from build123d import *

# Parameters (mm, degrees)
F0_R     = 3
F1_DEPTH = 3.95
F0_R_2   = 2.499
F2_DEPTH = 3.45
F3_R     = 3.69999
F4_R     = 3.7


# Not quite as in the source:
# - a fillet or chamfer is up to 0.001 mm smaller than in the source, because OpenCascade refuses the exact size


with BuildPart() as f1:
    # F0 (on Front) → F1 (new body, symmetric)
    with BuildSketch(Plane.XZ):
        Polygon((19.7, 0), (-19.7, 0), (-19.7, -23.4), (-12.3, -23.4), (-12.3, -7.4), (19.7, -7.4), align=None)
        with Locations((-16, -19.7)):
            Circle(F0_R, mode=Mode.SUBTRACT)
        with Locations((-16, -11.7)):
            Circle(F0_R, mode=Mode.SUBTRACT)
        with Locations((-16, -3.7)):
            Circle(F0_R, mode=Mode.SUBTRACT)
        with Locations((-8, -3.7)):
            Circle(F0_R, mode=Mode.SUBTRACT)
        with Locations((0, -3.7)):
            Circle(F0_R, mode=Mode.SUBTRACT)
        with Locations((8, -3.7)):
            Circle(F0_R, mode=Mode.SUBTRACT)
        with Locations((16, -3.7)):
            Circle(F0_R, mode=Mode.SUBTRACT)
    extrude(amount=F1_DEPTH, both=True)

    # F0 (on Front) → F2 (join, symmetric)
    with BuildSketch(Plane.XZ):
        with Locations((16, -3.7)):
            Circle(F0_R)
        with Locations((16, -3.7)):
            Circle(F0_R_2, mode=Mode.SUBTRACT)
        with Locations((8, -3.7)):
            Circle(F0_R)
        with Locations((8, -3.7)):
            Circle(F0_R_2, mode=Mode.SUBTRACT)
        with Locations((0, -3.7)):
            Circle(F0_R)
        with Locations((0, -3.7)):
            Circle(F0_R_2, mode=Mode.SUBTRACT)
        with Locations((-8, -3.7)):
            Circle(F0_R)
        with Locations((-8, -3.7)):
            Circle(F0_R_2, mode=Mode.SUBTRACT)
        with Locations((-16, -3.7)):
            Circle(F0_R)
        with Locations((-16, -3.7)):
            Circle(F0_R_2, mode=Mode.SUBTRACT)
        with Locations((-16, -19.7)):
            Circle(F0_R)
        with Locations((-16, -19.7)):
            Circle(F0_R_2, mode=Mode.SUBTRACT)
        with Locations((-16, -11.7)):
            Circle(F0_R)
        with Locations((-16, -11.7)):
            Circle(F0_R_2, mode=Mode.SUBTRACT)
    extrude(amount=F2_DEPTH, both=True)

    # F3 (radius 3.7 in the source; OpenCascade refuses exactly that, so slightly less here)
    f3_edges = [f1.edges().sort_by_distance(p)[0] for p in [
        (19.7, 0, 0),
        (19.7, 0, -7.4),
        (-12.3, 0, -23.4),
        (-19.7, 0, -23.4),
    ]]
    fillet(f3_edges, radius=F3_R)

    # F4
    f4_edges = [f1.edges().sort_by_distance(p)[0] for p in [
        (-19.7, 0, 0),
    ]]
    fillet(f4_edges, radius=F4_R)


solid = f1.part
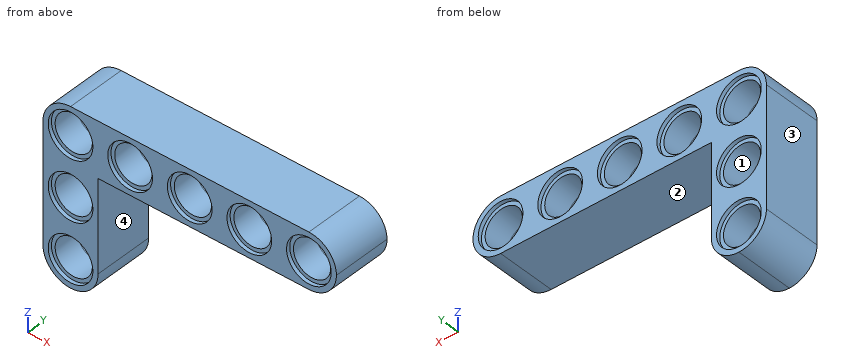
Could you check a few things on this model? Use its own coordinates, in mm. Face numbers are marked on the shaded views. Round coordinates to 2 decimals unless told otherwise and drop trailing zeros. Order: outer loops, then holes, each group sorted by start corner. A loop starts at its lowest first (then second) coordinate and runs counter-clockwise, first axis right, second up.
(1) I'm going to push flat-ended pins straight in: pin 1 (5.5 mm diameter, centred on x = -8, z = -3.7, fed in from +Y); pin 2 (1 mm diameter, centred on x = -6, y = 1, fed in from -Z); pin 3 (5.5 mm diameter, centred on x = -16, z = -19.7, fed in from -Y). Where does each tip first touch, or does it pass through?
Response values:
pin 1: stops at y = 3.45
pin 2: stops at z = -7.4
pin 3: stops at y = -3.45
(2) Please list where these lines run through material, in increasing order: line 1 along X through (y, z) = (1.5, -3.5); line 2 along Z through (x, y) = (-16, 2.3); line 3 along X through (y, z) = (-0.25, -5).
Response values:
line 1: x = -19.69 to -18.49, -13.51 to -10.49, -5.51 to -2.49, 2.49 to 5.51, 10.49 to 13.51, 18.49 to 19.69
line 2: z = -23.4 to -22.2, -17.2 to -14.2, -9.2 to -6.2, -1.2 to 0
line 3: x = -19.7 to -18.13, -13.87 to -10.13, -5.87 to -2.13, 2.13 to 5.87, 10.13 to 13.87, 18.13 to 19.46
(3) Imagine slicing it at A-A (x = -8). Write out the boundary of the cut face in (y, z), plus the area to 3 significant figures.
Response values:
outline: (-3.95, -7.4) - (3.95, -7.4) - (3.95, -6.7) - (3.45, -6.7) - (3.45, -6.2) - (-3.45, -6.2) - (-3.45, -6.7) - (-3.95, -6.7) - close; (-3.95, -0.7) - (-3.45, -0.7) - (-3.45, -1.2) - (3.45, -1.2) - (3.45, -0.7) - (3.95, -0.7) - (3.95, 0) - (-3.95, 0) - close
area: 18.0 mm2
(4) If we mould it in two halves opening along X, with no side actions, what happens to the marked faces 1, 2, 3 and 4? For each: released by +X, released by -X, zero draft, split by the parting line, or undercut.
Response values:
face 1: undercut
face 2: zero draft
face 3: released by -X
face 4: released by +X
(5) Imagine slicing it at D-D (x = 12.5). Write out the boundary of the cut face in (y, z).
Response values:
outline: (-3.95, -7.4) - (3.95, -7.4) - (3.95, 0) - (-3.95, 0) - close
(6) Imagine slicing it at B-B (y = 2.75). Count the separate pieces of the cut face and the enclosed holes in it, plus the area to 3 significant figures.
Response values:
separate pieces: 1
enclosed holes: 7
area: 258 mm2
(7) Imagine slicing it at C-C (z = -11.7). Write out the boundary of the cut face in (x, y).
Response values:
outline: (-19.7, -3.95) - (-19, -3.95) - (-19, -3.45) - (-18.5, -3.45) - (-18.5, 3.45) - (-19, 3.45) - (-19, 3.95) - (-19.7, 3.95) - close; (-13.5, -3.45) - (-13, -3.45) - (-13, -3.95) - (-12.3, -3.95) - (-12.3, 3.95) - (-13, 3.95) - (-13, 3.45) - (-13.5, 3.45) - close
